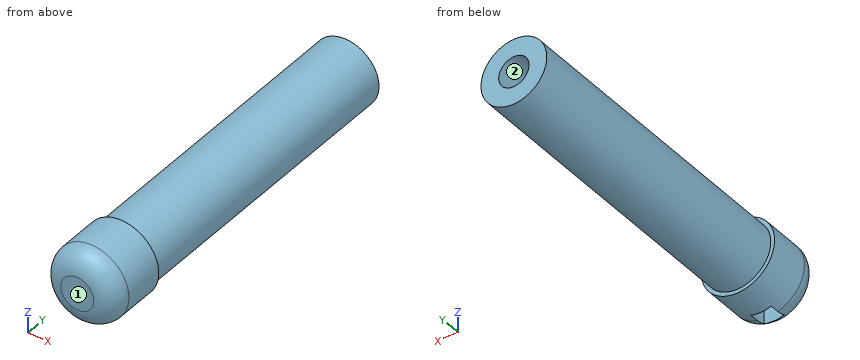
from build123d import *

# Parameters (mm, degrees)
SKETCH1_R                      = 6.5
BOSS_EXTRUDE1_DEPTH            = 60
SKETCH2_R                      = 3
INNER_CHAMBER_DEPTH            = 52.5
SKETCH4_R                      = 7.25
BOSS_EXTRUDE2_DEPTH            = 10
SKETCH5_R                      = 7.25
BOSS_EXTRUDE3_DEPTH            = 2
FILLET3_SIZE                   = 4
CUT_EXTRUDE2_REACH             = 62.87
SKETCH6_W                      = 4
SKETCH6_H                      = 3.5
CUT_EXTRUDE2_DIRECTION_2_DEPTH = 5


with BuildPart() as part:
    # Sketch1 → Boss-Extrude1 (new body)
    with BuildSketch(Plane(origin=(0, 0, 0), x_dir=(1, 0, 0), z_dir=(0, 1, 0))):
        with Locations(Location((0, 0, 0), (0, 0, 270))):
            Circle(SKETCH1_R)
    extrude(amount=BOSS_EXTRUDE1_DEPTH)

    # Sketch2 → Inner Chamber (cut)
    with BuildSketch(Plane(origin=(0, 60, 0), x_dir=(1, 0, 0), z_dir=(0, 1, 0))):
        with Locations(Location((0, 0, 0), (0, 0, 270))):
            Circle(SKETCH2_R)
    extrude(amount=-INNER_CHAMBER_DEPTH, mode=Mode.SUBTRACT)

    # Sketch4 → Boss-Extrude2 (add)
    with BuildSketch(Plane.XZ):
        with Locations(Location((0, 0, 0), (0, 0, 270))):
            Circle(SKETCH4_R)
    extrude(amount=BOSS_EXTRUDE2_DEPTH)

    # Sketch5 → Boss-Extrude3 (add)
    with BuildSketch(Plane.XZ.offset(10)):
        with Locations(Location((0, 0, 0), (0, 0, 270))):
            Circle(SKETCH5_R)
    extrude(amount=BOSS_EXTRUDE3_DEPTH)

    # Fillet3
    # a fillet whose section is not a circle: 4 mm, written as the material it takes off along each edge
    with BuildSketch(Plane(origin=(0, -12, 0), x_dir=(0, 0, -1), z_dir=(-1, 0, 0))) as fillet3_piece_1:
        with BuildLine():
            Bezier((7.25, -FILLET3_SIZE), (7.25, 0), (7.25 - FILLET3_SIZE, 0), weights=[1, 0.666666667, 1])
            Line((7.25 - FILLET3_SIZE, 0), (7.25, 0))
            Line((7.25, 0), (7.25, -FILLET3_SIZE))
        make_face()
    revolve(axis=Axis((0, -12, 0), (0, -1, 0)), mode=Mode.SUBTRACT)

    # Sketch6 → Cut-Extrude2 (cut, up to next)
    with BuildSketch(Plane.XY, mode=Mode.PRIVATE) as cut_extrude2_sk1:
        with Locations((0, -8)):
            Rectangle(SKETCH6_W, SKETCH6_H)
    cut_extrude2_tool1 = extrude(cut_extrude2_sk1.sketch, amount=-CUT_EXTRUDE2_REACH, mode=Mode.PRIVATE) & part.part
    add(cut_extrude2_tool1.solids().sort_by_distance((0, -8, 0))[0], mode=Mode.SUBTRACT)

    # Sketch6 → Cut-Extrude2 direction 2 (cut)
    with BuildSketch(Plane.XY):
        with Locations((0, -8)):
            Rectangle(SKETCH6_W, SKETCH6_H)
    extrude(amount=CUT_EXTRUDE2_DIRECTION_2_DEPTH, mode=Mode.SUBTRACT)


solid = part.part
Geometry check sheet. Reference: the model listing, model coordinates, mm. Face numbers are marked on the shaded views. A direction names the side the tool comes from. Give positions to 0.01 mm unless a question says otherwise; leave off trailing zeros. Loops run counter-clockwise (first coordinate to the right, second up) from the corner with the lowest first, then second, coordinate; pieces in that order, holes last. Notation, with made-up numbers: (9.5, -37.75) -> (35.5, -37.75) arc R8 cw to (35.5, -23.75) -> close; hole circle Ø2 at (86, 37.5). An arc over 180 degrees is marked (long way). Answer in a Markdown table with one row per item. Add a question column.
1) Gauge pin test, flat ends, axial feed: P1, Ø6, axis at x = -2, y = 19.5, coming from the +Z side; P2, Ø3, axis at x = -4, y = 42, coming from the -Z side; P3, Ø4, axis at x = 5, y = 3.5, coming from the +Z side; P4, Ø3, axis at x = 1, z = -1.5, coming from the +Y side. Record the tip position at first contact, or that the pin passes through.
2) Cross-section at B-B on y = 51.5. Record the boundary of the cut face in (x, z).
3) Material ranges on probe 1 along Y at (x, z) = (-1.75, -3); probe 2 along X at (y, z) = (24.5, 0); probe 3 along X at (y, z) = (34, 2.5), recorded low to high. Write a range as from..to.
4) Set-up check for the marked faces 1 and 2: record each of +Z, -Z, +X, -X, +Y, -Y from which the full face is reachable in a straight line by a thin tool's end or side.
5) Cross-section at A-A on y = 2. Record the boundary of the cut face in (x, z), and give its area (3 significant figures).
Outcome:
| question | item | result |
|---|---|---|
| 1 | P1 | stops at z = 6.5 |
| 1 | P2 | stops at z = -6 |
| 1 | P3 | stops at z = 5.77 |
| 1 | P4 | stops at y = 60 |
| 2 | outline | circle Ø13 at (0, 0); hole circle Ø6 at (0, 0) |
| 3 | probe 1 | y = -11.99..-9.75, -6.25..60 |
| 3 | probe 2 | x = -6.5..-3, 3..6.5 |
| 3 | probe 3 | x = -6..-1.66, 1.66..6 |
| 4 | face 1 | +Z, -Z, +X, -X, -Y |
| 4 | face 2 | +Y |
| 5 | outline | circle Ø13 at (0, 0) |
| 5 | area | 133 mm^2 |
